from build123d import *

# Parameters (mm, degrees)
F0_R     = 19.05
F1_DEPTH = 20.8662841469
F2_DEPTH = 40.5588373542


# Not quite as in the source:
# - the program builds the solid bodies; features that only make, move or delete a surface that nothing else refers to are left out


with BuildPart() as f1:
    # F0 (on Front) → F1 (new body)
    with BuildSketch(Plane.XZ):
        with BuildLine():
            Line((5.983272408, 44.0454645939), (0, 44.45))
            ThreePointArc((0, 44.45), (-44.45, 0), (0, -44.45))
            Line((0, -44.45), (5.983272408, -44.0454645939))
            ThreePointArc((5.983272408, -44.0454645939), (33.4795382177, -29.2390666871), (44.45, 0))
            ThreePointArc((44.45, 0), (33.4795382177, 29.2390666871), (5.983272408, 44.0454645939))
        make_face()
        Circle(F0_R, mode=Mode.SUBTRACT)
        with BuildLine():
            Line((142.0559377087, 34.8454470844), (5.983272408, 44.0454645939))
            ThreePointArc((5.983272408, 44.0454645939), (33.4795382177, 29.2390666871), (44.45, 0))
            ThreePointArc((44.45, 0), (33.4795382177, -29.2390666871), (5.983272408, -44.0454645939))
            Line((5.983272408, -44.0454645939), (142.0559377087, -34.8454470844))
            ThreePointArc((142.0559377087, -34.8454470844), (104.775, 0), (142.0559377087, 34.8454470844))
        make_face()
        with BuildLine():
            ThreePointArc((174.625, 0), (165.2150617232, 23.8482127268), (142.0559377087, 34.8454470844))
            ThreePointArc((142.0559377087, 34.8454470844), (104.775, 0), (142.0559377087, -34.8454470844))
            ThreePointArc((142.0559377087, -34.8454470844), (165.2150617232, -23.8482127268), (174.625, 0))
        make_face()
        with Locations((139.7, 0)):
            Circle(F0_R, mode=Mode.SUBTRACT)
    extrude(amount=-F1_DEPTH)

    # F0 (on Front) → F2 (join)
    with BuildSketch(Plane.XZ):
        with BuildLine():
            Line((5.983272408, 44.0454645939), (0, 44.45))
            ThreePointArc((0, 44.45), (-44.45, 0), (0, -44.45))
            Line((0, -44.45), (5.983272408, -44.0454645939))
            ThreePointArc((5.983272408, -44.0454645939), (33.4795382177, -29.2390666871), (44.45, 0))
            ThreePointArc((44.45, 0), (33.4795382177, 29.2390666871), (5.983272408, 44.0454645939))
        make_face()
        Circle(F0_R, mode=Mode.SUBTRACT)
    extrude(amount=-F2_DEPTH)


solid = f1.part
Part model, mm, in its own coordinate system. Give positions to 0.01 mm unless a question says otherwise; leave off trailing zeros. Order: outer loops, then holes, each group sorted by start corner. A loop starts at its lowest first (then second) coordinate and runs counter-clockwise, first axis right, second up. Notation, with made-up numbers: (41.5, 2.25) -> (80.5, 2.25) arc R19 cw to (80.5, 17.25) -> close; hole circle Ø2 at (44.5, -11.75). An arc over 180 degrees is marked (long way). Use one line per item in the form item = value.
(1) Saw through at D-D (y = 35.5). Write the cut outline in (x, z), then the cut area to 3 significant figures.
Solution:
outline = (0, -44.45) -> (5.98, -44.05) arc R44.45 ccw to (5.98, 44.05) -> (0, 44.45) arc R44.45 ccw to start; hole circle Ø38.1 at (0, 0)
area = 5,070 mm²
(2) Flat gauge pins, fed straight in: P1, Ø10, axis at y = 34, z = 8.5, coming from the +X side; P2, Ø8, axis at y = 20.5, z = -25.5, coming from the +X side; P3, Ø4, axis at x = 66, y = 21.5, coming from the -Z side; P4, Ø1, axis at x = 20, z = -22.5, coming from the -Y side. Where does each tip first touch, or does it go through?
Solution:
P1 = 44.31
P2 = 167.22
P3 = -40.12
P4 = 0
(3) Saw through at C-C (x = 140). Write the cut outline in (y, z).
Solution:
outline = (0, -34.98) -> (20.87, -34.98) -> (20.87, -19.05) -> (0, -19.05) -> close; (0, 19.05) -> (20.87, 19.05) -> (20.87, 34.98) -> (0, 34.98) -> close
(4) Pull direction Z, two halves, no side cores. Call faces 1 (the face through (157.87, 10.29, 5.72)), 2 (the face through (-44.44, 20, 0.98)), 3 (the face through (64, 0, 1)): +Z half, -Z half, draft (parallel to the pull), parting line (faces both ways), or undercut.
Solution:
face_1 = undercut
face_2 = parting line
face_3 = draft
(5) Saw through at A-A (y = 13). Write the cut outline in (x, z) (3 decimals).
Solution:
outline = (0, -44.45) -> (142.056, -34.845) arc R34.925 ccw to (142.056, 34.845) -> (0, 44.45) arc R44.45 ccw to start; hole circle Ø38.1 at (0, 0); hole circle Ø38.1 at (139.7, 0)
(6) Drill centre lines: line 1 (Y direction, x = 110, z = 35); line 2 (X direction, y = 16, z = 15.5); line 3 (Z direction, x = 139, y = 13). Where is each one in solid material? Low to high. Write a range as from..to.
Solution:
line_1 = 0..20.87
line_2 = -41.66..-11.07, 11.07..128.63, 150.77..171
line_3 = -35.05..-19.04, 19.04..35.05
(7) Saw through at B-B (z = -7.5). Write the cut outline in (x, y).
Solution:
outline = (-43.81, 0) -> (-17.51, 0) -> (-17.51, 40.56) -> (-43.81, 40.56) -> close; (17.51, 0) -> (122.19, 0) -> (122.19, 20.87) -> (43.81, 20.87) -> (43.81, 40.56) -> (17.51, 40.56) -> close; (157.21, 0) -> (173.81, 0) -> (173.81, 20.87) -> (157.21, 20.87) -> close
